The model under review builds one solid part; all positions refer to its coordinate system, in mm. Face numbers are marked on the shaded views. A direction names the side the tool comes from. Coordinates: 2 decimals unless noted, no trailing zeros. Write each loop counter-clockwise with the first axis right and the second up, starting at its lowest first coordinate (ties: lowest second). Pieces come first, ordered by that corner, then holes. Notation, with made-up numbers: (-22.75, 37.5) - (-6.75, 37.5) arc R11 ccw to (-6.75, 45.5) - close; hole circle Ø7 at (24.5, 44.5). An arc over 180 degrees is marked (long way). Put each result on its own line as item: value. Start each with the question number.
Item 1: Consider section A-A on z = 0. Give the boundary of the cut face in (x, y), then the cut area to 3 significant figures.
Item 2: Mouldability with a two-part tool opening along Z and no side actions: class the marked faces 4, 5, 6 and 7 as pulls with the +Z half, pulls with the -Z half, needs draft (parallel to the pull), parting line crosses it, or undercut.
Item 3: For pin 1 (4 mm diameter, centred on x = -30, z = 69.5, fed in from +Y); pin 2 (13.5 mm diameter, centred on x = -80, y = 49.5, fed in from +Z); pin 3 (17 mm diameter, centred on x = 79.92, z = 79.92, fed in from +Y); pin 4 (1.5 mm diameter, centred on y = 58, z = -1, fed in from -X), all flat-tipped, find the tip position at first contact; note any pin that passes through.
Item 4: Consider section D-D on y = 40. Give the boundary of the cut face in (x, z), then the cut area to 3 significant figures.
Item 5: Machinability: for the marked faces 1, 2 and 3, which of the approach directions +Z, -Z, +X, -X, +Y, -Y give a long, thin tool a straight path to every point of the face, cutting with its end or side? Answer none if there is none.
Item 6: Consider section C-C on y = 59.5. Give the boundary of the cut face in (x, z).
Item 7: Consider section B-B on x = 0. Give the boundary of the cut face in (y, z).
Item 8: To check wall thickness, follow L1, parallel to X at y = 74.5, z = 59; L2, parallel to X at y = 57.5, z = 31.5; L3, parallel to Y at x = -60.5, z = 67.5. State the ranges of each line that lie inside material, in increasing order. Write a range as [from, to].
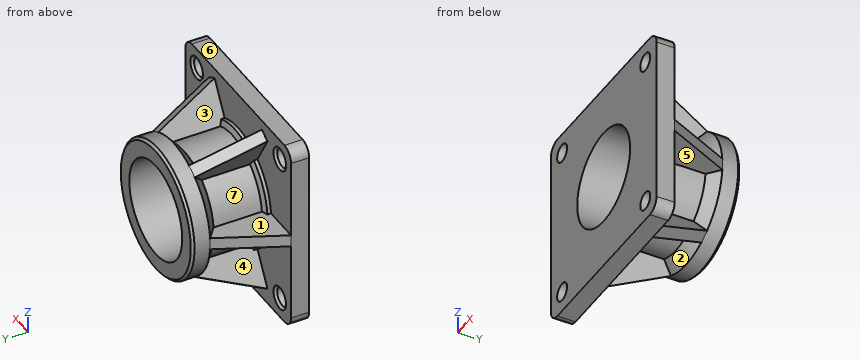
```python
from build123d import *

# Parameters (mm, degrees)
BASE_SKETCH_W               = 203.2
BASE_SKETCH_H               = 203.2
BASE_FEATURE_DEPTH          = 19.05
SHAFT_HOLE_SKETCH_R         = 50.8
SHAFT_HOLE_FEATURE_DEPTH    = 179.361745911
BASE_FILLET_R               = 12.7
BOLTING_HOLES_SKETCH_R      = 9.525
BOLTING_HOLES_FEATURE_DEPTH = 168.778102347
RIB_SUPPORT_FEATURE_REACH   = 180.362
RIB_SUPPORT_SKETCH_WALL_W   = 433.38819801
RIB_SUPPORT_SKETCH_WALL_H   = 12.7
RIB_SUPPORT_PATTERN_COUNT   = 6
CHAMFER1_SIZE               = 2.54


with BuildPart() as part:
    # Base Sketch → Base Feature (new body)
    with BuildSketch(Plane(origin=(0, 0, 0), x_dir=(1, 0, 0), z_dir=(0, 1, 0))):
        Rectangle(BASE_SKETCH_W, BASE_SKETCH_H)
    extrude(amount=BASE_FEATURE_DEPTH)

    # Shaft Housing Sketch → Shaft Housing Feature (revolve)
    with BuildSketch(Plane.XY, mode=Mode.PRIVATE) as shaft_housing_feature_sk:
        Polygon((63.5, 19.05), (63.5, 22.86), (57.15, 25.171210988), (57.15, 75.971210988), (69.85, 86.627776304), (69.85, 105.677776304), (50.8, 105.677776304), (50.8, 19.05), align=None)
    revolve(shaft_housing_feature_sk.sketch.rotate(Axis((0, 0, 0), (0, -1, 0)), 90), axis=Axis((0, 0, 0), (0, -1, 0)))

    # Shaft Hole Sketch → Shaft Hole Feature (cut, through all)
    with BuildSketch(Plane(origin=(0, 105.677776304, 0), x_dir=(1, 0, 0), z_dir=(0, 1, 0))):
        with Locations(Location((0, 0, 0), (0, 0, 270))):
            Circle(SHAFT_HOLE_SKETCH_R)
    extrude(amount=-SHAFT_HOLE_FEATURE_DEPTH, mode=Mode.SUBTRACT)

    # Base Fillet
    base_fillet_edges = [part.edges().sort_by_distance(p)[0] for p in [
        (-101.6, 9.525, -101.6),
        (101.6, 9.525, -101.6),
        (101.6, 9.525, 101.6),
        (-101.6, 9.525, 101.6),
    ]]
    fillet(base_fillet_edges, radius=BASE_FILLET_R)

    # Bolting Holes Sketch → Bolting Holes Feature (cut, through all)
    with BuildSketch(Plane(origin=(0, 19.05, 0), x_dir=(1, 0, 0), z_dir=(0, 1, 0))):
        with Locations(Location((-79.919743879, 79.919743879, 0), (0, 0, 270))):
            Circle(BOLTING_HOLES_SKETCH_R)
        with Locations(Location((79.919743879, 79.919743879, 0), (0, 0, 270))):
            Circle(BOLTING_HOLES_SKETCH_R)
        with Locations(Location((79.919743879, -79.919743879, 0), (0, 0, 270))):
            Circle(BOLTING_HOLES_SKETCH_R)
        with Locations(Location((-79.919743879, -79.919743879, 0), (0, 0, 270))):
            Circle(BOLTING_HOLES_SKETCH_R)
    extrude(amount=-BOLTING_HOLES_FEATURE_DEPTH, mode=Mode.SUBTRACT)

    # Rib Support Sketch wall → Rib Support Feature (add, up to next)
    with BuildSketch(Plane(origin=(-85.725, 52.838888152, 0), x_dir=(-0.425234379412, -0.905083268305, 0), z_dir=(0.905083268305, -0.425234379412, 0)), mode=Mode.PRIVATE) as rib_support_feature_sk1:
        Rectangle(RIB_SUPPORT_SKETCH_WALL_W, RIB_SUPPORT_SKETCH_WALL_H)
    rib_support_feature_tool1 = extrude(rib_support_feature_sk1.sketch, amount=RIB_SUPPORT_FEATURE_REACH, mode=Mode.PRIVATE) - part.part
    rib_support_feature = rib_support_feature_tool1.solids().sort_by_distance((-85.725, 52.838888152, 0))[0]
    add(rib_support_feature)

    # Rib Support Pattern: Rib Support Feature ×6 about axis
    rib_support_pattern_axis = Axis((0, 0, 0), (0, 1, 0))
    for i in range(1, RIB_SUPPORT_PATTERN_COUNT):
        add(rib_support_feature.rotate(rib_support_pattern_axis, i * 360 / RIB_SUPPORT_PATTERN_COUNT))

    # Chamfer1
    chamfer1_edges = [part.edges().sort_by_distance(p)[0] for p in [
        (0, 105.677776304, -69.85),
        (-79.919743879, 19.05, -89.444743879),
        (79.919743879, 19.05, -89.444743879),
        (79.919743879, 19.05, 70.394743879),
        (-79.919743879, 19.05, 70.394743879),
    ]]
    chamfer(chamfer1_edges, length=CHAMFER1_SIZE)


solid = part.part
```
Report:
1. outline: (-101.6, 0) - (-50.8, 0) - (-50.8, 105.68) - (-67.31, 105.68) - (-69.85, 103.14) - (-69.85, 86.63) - (-101.6, 19.05) - close; (50.8, 0) - (101.6, 0) - (101.6, 19.05) - (69.85, 86.63) - (69.85, 103.14) - (67.31, 105.68) - (50.8, 105.68) - close
1. area: 7,380 mm²
2. face 4: undercut
2. face 5: pulls with the -Z half
2. face 6: pulls with the +Z half
2. face 7: undercut
3. pin 1: y = 19.05
3. pin 2: z = 6.35
3. pin 3: through
3. pin 4: x = -83.65
4. outline: (-91.76, -6.35) - (-56.8, -6.35) arc R57.15 ccw to (-33.9, -46.01) - (-51.38, -76.29) - (-40.38, -82.64) - (-22.9, -52.36) arc R57.15 ccw to (22.9, -52.36) - (40.38, -82.64) - (51.38, -76.29) - (33.9, -46.01) arc R57.15 ccw to (56.8, -6.35) - (91.76, -6.35) - (91.76, 6.35) - (56.8, 6.35) arc R57.15 ccw to (33.9, 46.01) - (51.38, 76.29) - (40.38, 82.64) - (22.9, 52.36) arc R57.15 ccw to (-22.9, 52.36) - (-40.38, 82.64) - (-51.38, 76.29) - (-33.9, 46.01) arc R57.15 ccw to (-56.8, 6.35) - (-91.76, 6.35) - close; hole circle Ø101.6 at (0, 0)
4. area: 4,800 mm²
5. face 1: +Z, -X
5. face 2: -Z
5. face 3: +Z
6. outline: (-82.6, -6.35) - (-56.8, -6.35) arc R57.15 ccw to (-33.9, -46.01) - (-46.8, -68.35) - (-35.8, -74.7) - (-22.9, -52.36) arc R57.15 ccw to (22.9, -52.36) - (35.8, -74.7) - (46.8, -68.35) - (33.9, -46.01) arc R57.15 ccw to (56.8, -6.35) - (82.6, -6.35) - (82.6, 6.35) - (56.8, 6.35) arc R57.15 ccw to (33.9, 46.01) - (46.8, 68.35) - (35.8, 74.7) - (22.9, 52.36) arc R57.15 ccw to (-22.9, 52.36) - (-35.8, 74.7) - (-46.8, 68.35) - (-33.9, 46.01) arc R57.15 ccw to (-56.8, 6.35) - (-82.6, 6.35) - close; hole circle Ø101.6 at (0, 0)
7. outline: (0, -101.6) - (19.05, -101.6) - (19.05, -63.5) - (22.86, -63.5) - (25.17, -57.15) - (75.97, -57.15) - (86.63, -69.85) - (103.14, -69.85) - (105.68, -67.31) - (105.68, -50.8) - (0, -50.8) - close; (0, 50.8) - (105.68, 50.8) - (105.68, 67.31) - (103.14, 69.85) - (86.63, 69.85) - (75.97, 57.15) - (25.17, 57.15) - (22.86, 63.5) - (19.05, 63.5) - (19.05, 101.6) - (0, 101.6) - close
8. L1: [-41.4, -26.73], [26.73, 41.4]
8. L2: [-47.69, -39.85], [39.85, 47.69]
8. L3: [0, 19.05]
